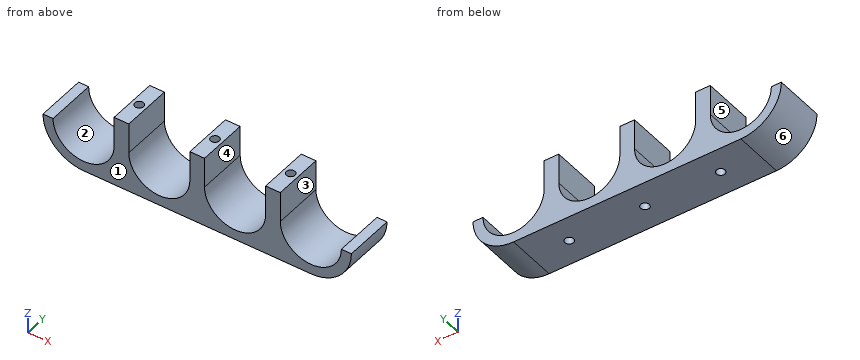
```python
from build123d import *

# Parameters (mm, degrees)
BOSS_EXTRUDE1_DEPTH  = 15
M2_CLEARANCE_HOLE2_D = 2.6


with BuildPart() as part:
    # Sketch1 → Boss-Extrude1 (new body)
    with BuildSketch(Plane(origin=(0, 0, 0), x_dir=(1, 0, 0), z_dir=(0, 1, 0))):
        with BuildLine():
            Line((2.2, 0), (2.2, -9.15))
            Line((2.2, -9.15), (-2.2, -9.15))
            Line((-2.2, -9.15), (-2.2, 0))
            ThreePointArc((-2.2, 0), (-11.35, 9.15), (-20.5, 0))
            Line((-20.5, 0), (-20.5, -9.15))
            Line((-20.5, -9.15), (-24.9, -9.15))
            Line((-24.9, -9.15), (-24.9, 0))
            ThreePointArc((-24.9, 0), (-34.05, 9.15), (-43.2, 0))
            Line((-43.2, 0), (-46.2, 0))
            ThreePointArc((-46.2, 0), (-42.641347391, 8.591347391), (-34.05, 12.15))
            Line((-34.05, 12.15), (34.05, 12.15))
            ThreePointArc((34.05, 12.15), (42.641347391, 8.591347391), (46.2, 0))
            Line((46.2, 0), (43.2, 0))
            ThreePointArc((43.2, 0), (34.05, 9.15), (24.9, 0))
            Line((24.9, 0), (24.9, -9.15))
            Line((24.9, -9.15), (20.5, -9.15))
            Line((20.5, -9.15), (20.5, 0))
            ThreePointArc((20.5, 0), (11.35, 9.15), (2.2, 0))
        make_face()
    extrude(amount=BOSS_EXTRUDE1_DEPTH)

    # M2 Clearance Hole2 (through all)
    with Locations(Plane(origin=(0, 0, -12.15), x_dir=(-1, 0, 0), z_dir=(0, 0, -1))):
        with Locations((0, 7.5), (-22.7, 7.5), (22.7, 7.5)):
            Hole(M2_CLEARANCE_HOLE2_D / 2)


solid = part.part
```
Model file for the job. Use its own axes, mm. Face numbers are marked on the shaded views. A direction names the side the tool comes from. Coordinates: 2 decimals unless noted, no trailing zeros. Order: outer loops, then holes, each group sorted by start corner. A loop starts at its lowest first (then second) coordinate and runs counter-clockwise, first axis right, second up. Notation, with made-up numbers: (47, 69) -> (69, 69) arc R12 ccw to (69, 90) -> close; hole circle Ø1 at (-19, 65.5). An arc over 180 degrees is marked (long way). Answer as a JSON object with one key per item and string values. Group by question number.
1) Flat gauge pins, fed straight in: pin 1 (7.5 mm diameter, centred on y = 5, z = 2.5, fed in from -X); pin 2 (3.5 mm diameter, centred on x = -44.5, y = 7.5, fed in from +Z); pin 3 (1 mm diameter, centred on y = 4, z = -8.5, fed in from -X); pin 4 (5 mm diameter, centred on y = 4, z = -10, fed in from -X). Where does each tip first touch, or does it go through?
2) Cut at B-B, the plane z = 1.5. Write the cut outline in (x, y).
3) Pull direction X, two halves, no side cores. Call the marked faces 1, 2 and 3: +X half, -X half, draft (parallel to the pull), parting line (faces both ways), or undercut.
4) Cut at A-A, the plane y = 7.5. Count the separate pieces of the cut face and the enclosed holes in it, then the cut area to 3 significant figures.
5) Cut at D-D, the plane z = -6.25. Write the cut outline in (x, y), then the cut area to 3 significant figures.
6) Drill centre lines: L1, parallel to X at y = 11, z = 6; L2, parallel to X at y = 14, z = -0.5; L3, parallel to Y at x = -22.7, z = -0.25. Where is each one in solid material? Low to high.
7) Which spindle directions (+Z, -Z, +X, -X, +Y, -Y) get a long thin tool onto all of the face, cutting with end or side? Do the marked faces 4, 5 and 6. Say none if no direction does.
8) Cut at C-C, the plane x = 22.7. Write the cut outline in (y, z).
Check values:
{
 "1": {"pin 1": "stops at x = -46.2", "pin 2": "stops at z = 0", "pin 3": "stops at x = -43.19", "pin 4": "stops at x = -43.61"},
 "2": {"outline": "(-24.9, 0) -> (-20.5, 0) -> (-20.5, 15) -> (-24.9, 15) -> close; (-2.2, 0) -> (2.2, 0) -> (2.2, 15) -> (-2.2, 15) -> close; (20.5, 0) -> (24.9, 0) -> (24.9, 15) -> (20.5, 15) -> close; hole circle Ø2.6 at (-22.7, 7.5); hole circle Ø2.6 at (0, 7.5); hole circle Ø2.6 at (22.7, 7.5)"},
 "3": {"face 1": "draft", "face 2": "undercut", "face 3": "+X half"},
 "4": {"separate pieces": "4", "enclosed holes": "0", "area": "488 mm²"},
 "5": {"outline": "(-44.47, 0) -> (-40.73, 0) -> (-40.73, 15) -> (-44.47, 15) -> close; (-27.37, 0) -> (-18.03, 0) -> (-18.03, 15) -> (-27.37, 15) -> close; (-4.67, 0) -> (4.67, 0) -> (4.67, 15) -> (-4.67, 15) -> close; (18.03, 0) -> (27.37, 0) -> (27.37, 15) -> (18.03, 15) -> close; (40.73, 0) -> (44.47, 0) -> (44.47, 15) -> (40.73, 15) -> close; hole circle Ø2.6 at (-22.7, 7.5); hole circle Ø2.6 at (0, 7.5); hole circle Ø2.6 at (22.7, 7.5)", "area": "516 mm²"},
 "6": {"L1": "x = -24.9 to -20.5, -2.2 to 2.2, 20.5 to 24.9", "L2": "x = -46.19 to -43.19, -24.91 to -20.49, -2.21 to 2.21, 20.49 to 24.91, 43.19 to 46.19", "L3": "y = 0 to 6.2, 8.8 to 15"},
 "7": {"face 4": "+Z, +Y, -Y", "face 5": "+Z, -X, +Y, -Y", "face 6": "-Z, -X, +Y, -Y"},
 "8": {"outline": "(0, -12.15) -> (6.2, -12.15) -> (6.2, 9.15) -> (0, 9.15) -> close; (8.8, -12.15) -> (15, -12.15) -> (15, 9.15) -> (8.8, 9.15) -> close"}
}
